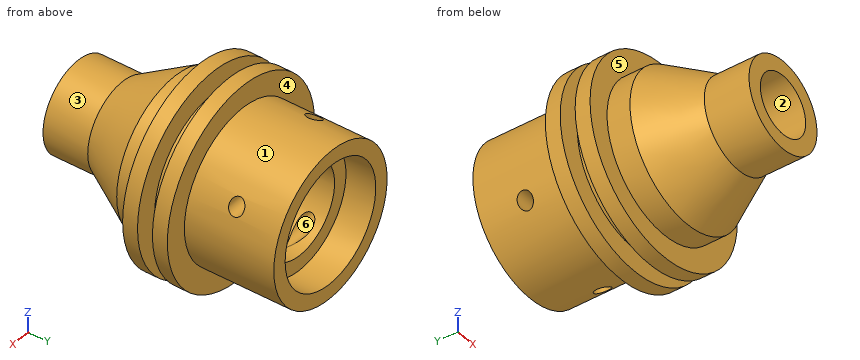
Autodesk Inventor part; units mm, degrees
ref_plane "Work Plane1" through (0, 14, 3) normal (0, 0, -1) x (-1, 0, 0)
ref_plane "YZ Plane" through (0, 0, 0) normal (1, 0, 0) x (0, 1, 0)
ref_plane "XZ Plane" through (0, 0, 0) normal (0, 1, 0) x (-1, 0, 0)
sketch "Sketch1" plane through (0, 0, 0) normal (0, 0, 1) x (1, 0, 0)
  line L0 (2, 0) -> (2, 7)
  line L1 (2, 7) -> (3, 8.7321)
  line L2 (3, 8.7321) -> (3, 15)
  line L3 (3, 15) -> (4, 15)
  line L4 (4, 15) -> (4, 17)
  line L5 (4, 17) -> (5, 17)
  line L6 (5, 17) -> (5, 11)
  line L7 (5, 11) -> (6.5, 11)
  line L8 (6.5, 11) -> (6.5, 10)
  line L9 (6.5, 10) -> (5, 10)
  line L10 (5, 10) -> (5, 9)
  line L11 (5, 9) -> (6.5, 9)
  line L12 (6.5, 9) -> (6.5, 8)
  line L13 (6.5, 8) -> (5, 8)
  line L14 (5, 8) -> (5, 6.4641)
  line L15 (5, 6.4641) -> (3, 3)
  line L16 (3, 3) -> (3, 0)
  line L17 (3, 0) -> (2, 0)
  line L18 (0, -3.4) -> (0, 20.4)
  point P0 (0, 0)
  dimension "d0" = 7
  dimension "d1" = 17
  dimension "d2" = 2
  dimension "d3" = 3
  dimension "d4" = 1
  dimension "d5" = 1
  dimension "d6" = 1
  dimension "d7" = 2
  dimension "d8" = 11
  dimension "d9" = 1.5
  dimension "d10" = 5
  dimension "d11" = 60
  dimension "d13" = 4
  dimension "d14" = 3
  dimension "d48" = 4
revolve "Revolution1" add sketch "Sketch1" angle 360 about axis through (0, -10, 0) along (0, 1, 0)
sketch "Sketch2" plane through (0, 0, 0) normal (1, 0, 0) x (0, 1, 0)
  line L0 (8.7321, 3) -> (15, 3)
  point P0 (0, 0)
  point P1 (14, 3)
  dimension "d15" = 1
  dimension "d35" = 3
ref_plane "Work Plane1" through (0, 14, 3) normal (0, 0, -1) x (-1, 0, 0)
sketch "Sketch4" plane through (0, 0, 0) normal (1, 0, 0) x (0, 1, 0)
  line L0 (11, 6.5) -> (11, -6.5)
  point P0 (0, 0)
  point P1 (14, 2.5)
  dimension "d36" = 3
  dimension "d37" = 2.5
hole "Hole3" at (0, 14, 2.5) direction (1, 0, 0) diameter 1 end through all
pattern_circular "Circular Pattern2" count 4 over 360 about axis through (0, -10, 0) along (0, 1, 0) of "Hole3"
properties part number "inner element" material "Brass, Soft Yellow"
The listing builds one solid part. Answer for the finished solid, in the listing's coordinates (mm). Face numbers are marked on the shaded views. A direction names the side the tool comes from. Coordinates: 2 decimals unless noted, no trailing zeros. Order: outer loops, then holes, each group sorted by start corner. A loop starts at its lowest first (then second) coordinate and runs counter-clockwise, first axis right, second up. Notation, with made-up numbers: M 62,18 L 76,18 A15 ccw 76,39 Z; hole C -6,-25.75 d1. An arc over 180 degrees is marked long. Answer as a JSON object with one key per item and string values. Group by question number.
1. Determine the mould class of the marked faces 4, 5 and 6 for opening direction Y: released by +Y, released by -Y, zero draft, split by the parting line, or undercut.
2. A tool of negligible diameter and unlimited length cuts with its end or side. For the marked faces 1, 2 and 3, from which of +Z, -Z, +X, -X, +Y, -Y can it reach the whole face along a straight path? Write none if from no direction.
3. Straight lines are drawn through the part: line 1 (X direction, y = 12.25, z = 0); line 2 (Y direction, x = -5.75, z = 0); line 3 (X direction, y = 2, z = 0). For each, find the intervals that lie inside material, in ascending order.
4. Section C-C on x = 2.5 is taken. State how many separate pieces and enclosed holes the cut face has, then the cut area to 3 significant figures.
5. Section A-A on y = 14 is taken. Write down the section's boundary in (x, z).
6. Flat-ended cylindrical pins translate along their axes: P1, Ø4, axis at x = -3.5, y = 2, coming from the +Z side; P2, Ø1.5, axis at x = 3.5, y = 12, coming from the -Z side; P3, Ø2, axis at x = 3.5, z = 2.5, coming from the -Y side. Find the tip coordinate at first contact, or state that the pin passes through.
7. Section B-B on z = 5.5 is taken. Write down the section's boundary in (x, y), then the cut area to 3 significant figures.
Values follow:
{
 "1": {"face 4": "released by +Y", "face 5": "released by -Y", "face 6": "undercut"},
 "2": {"face 1": "+Y", "face 2": "+Y, -Y", "face 3": "-Y"},
 "3": {"line 1": "-5 to -3, 3 to 5", "line 2": "8 to 9, 10 to 11", "line 3": "-3 to -2, 2 to 3"},
 "4": {"separate pieces": "2", "enclosed holes": "1", "area": "90.6 mm2"},
 "5": {"outline": "M -4.58,-2 L -2.24,-2 A3 cw -3,0 L -3,4 A5 ccw Z; M -4,-3 A5 ccw 2,-4.58 L 2,-2.24 A3 cw 0,-3 Z; M -2,2.24 A3 cw 0,3 L 4,3 A5 ccw -2,4.58 Z; M 2.24,2 A3 cw 3,0 L 3,-4 A5 ccw 4.58,2 Z"},
 "6": {"P1": "z = 2.6", "P2": "z = -4.18", "P3": "y = 3.52"},
 "7": {"outline": "M -3.46,8 L 3.46,8 L 3.46,9 L -3.46,9 Z; M -3.46,10 L 3.46,10 L 3.46,11 L -3.46,11 Z", "area": "13.9 mm2"}
}
